```python
from build123d import *

# Parameters (mm, degrees)
BOSS_EXTRUDE1_DEPTH = 63.5
SKETCH2_R           = 3.175
CUT_EXTRUDE1_DEPTH  = 127


with BuildPart() as part:
    # Sketch1 → Boss-Extrude1 (new, symmetric)
    with BuildSketch(Plane.XY):
        Polygon((6.500914077, 0), (-18.899085923, 0), (-18.899085923, 25.4), (-15.724085923, 25.4), (-15.724085923, 3.175), (6.500914077, 3.175), align=None)
    extrude(amount=BOSS_EXTRUDE1_DEPTH, both=True)

    # Sketch2 → Cut-Extrude1 (cut)
    with BuildSketch(Plane.ZY.offset(18.899085923)):
        with Locations((50.8, 12.7)):
            Circle(SKETCH2_R)
        with Locations(Location((-50.8, 12.7, 0), (0, 0, 270))):
            Circle(SKETCH2_R)
    extrude(amount=-CUT_EXTRUDE1_DEPTH, mode=Mode.SUBTRACT)


solid = part.part
```
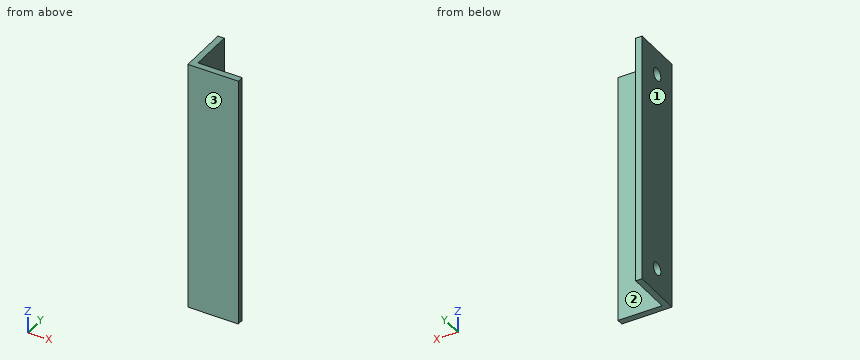
Could you check a few things on this model? Use its own coordinates, in mm. Face numbers are marked on the shaded views. Coordinates: 2 decimals unless noted, no trailing zeros. Order: outer loops, then holes, each group sorted by start corner. A loop starts at its lowest first (then second) coordinate and runs counter-clockwise, first axis right, second up. Notation, with made-up numbers: M -2,73.5 L 56,73.5 A24 cw 56,84.5 Z; hole C 31.25,19 d3. An arc over 180 degrees is marked long. Use one line per item in the form item = value. Start each with the question number.
1. For pin 1 (4 mm diameter, centred on y = 12.7, z = -50.8, fed in from +X); pin 2 (1.5 mm diameter, centred on y = 6, z = 46.5, fed in from +X); pin 3 (4 mm diameter, centred on x = -5, z = 10.5, fed in from +Y) (3 decimals), each with a flat end and sliding along its axis, tell me the tip position at first contact or that it passes through.
2. Suppose I cut it at A-A on z = -50.8. Write out the boundary of the cut face in (x, y) (3 decimals), then the cut area to 3 significant figures.
3. Suppose I cut it at B-B on y = 12.7. Write out the boundary of the cut face in (x, z) (3 decimals).
4. We'd pull the mould along Y, two halves only. Please class the marked faces 1, 2 and 3: +Y half, -Y half, draft (parallel to the pull), parting line (faces both ways), or undercut.
5. Suppose I cut it at C-C on x = 2.75. Write out the boundary of the cut face in (y, z) (3 decimals), then the cut area to 3 significant figures.
6. Suppose I cut it at D-D on z = 28. Write out the boundary of the cut face in (x, y) (3 decimals), then the cut area to 3 significant figures.
7. Please list where these lines run through material, in increasing order: line 1 (Y direction, x = -17.9, z = 50.8) (3 decimals); line 2 (Y direction, x = -10, z = -56) (3 decimals); line 3 (X direction, y = 17.75, z = 5.5).
Geometry says:
q1.pin_1 = through
q1.pin_2 = -15.72
q1.pin_3 = 3.175
q2.outline = M -18.899,0 L 6.501,0 L 6.501,3.175 L -15.724,3.175 L -15.724,9.525 L -18.899,9.525 Z; M -18.899,15.875 L -15.724,15.875 L -15.724,25.4 L -18.899,25.4 Z
q2.area = 131 mm^2
q3.outline = M -18.899,-63.5 L -15.724,-63.5 L -15.724,-53.975 L -18.899,-53.975 Z; M -18.899,-47.625 L -15.724,-47.625 L -15.724,47.625 L -18.899,47.625 Z; M -18.899,53.975 L -15.724,53.975 L -15.724,63.5 L -18.899,63.5 Z
q4.face_1 = draft
q4.face_2 = +Y half
q4.face_3 = -Y half
q5.outline = M 0,-63.5 L 3.175,-63.5 L 3.175,63.5 L 0,63.5 Z
q5.area = 403 mm^2
q6.outline = M -18.899,0 L 6.501,0 L 6.501,3.175 L -15.724,3.175 L -15.724,25.4 L -18.899,25.4 Z
q6.area = 151 mm^2
q7.line_1 = 0 to 9.525, 15.875 to 25.4
q7.line_2 = 0 to 3.175
q7.line_3 = -18.9 to -15.72
